from build123d import *

# Parameters (mm, degrees)
SKETCH003_R   = 2
PAD002_DEPTH  = 10
SKETCH_R      = 7
PAD_DEPTH     = 45
SKETCH001_W   = 100
SKETCH001_H   = 10
PAD001_DEPTH  = 5
FILLET_R      = 4.99
SKETCH002_W   = 3
SKETCH002_H   = 13.521623
SKETCH002_H_2 = 14.821778
SKETCH002_H_3 = 14.691763
POCKET_DEPTH  = 4


with BuildPart() as pad002:
    # Sketch003 → Pad002 (new body, symmetric)
    with BuildSketch(Plane(origin=(0, 0, -4), x_dir=(0, 0, -1), z_dir=(1, 0, 0))):
        Circle(SKETCH003_R)
    extrude(amount=PAD002_DEPTH, both=True)


with BuildPart() as cut:
    # Sketch → Pad (new body)
    with BuildSketch(Plane.XY):
        Circle(SKETCH_R)
    extrude(amount=-PAD_DEPTH)

    # Cut: cut Pad002
    add(pad002.part, mode=Mode.SUBTRACT)


with BuildPart() as obj1:
    # Sketch001 → Pad001 (new body, symmetric)
    with BuildSketch(Plane.XY.offset(-45)):
        Rectangle(SKETCH001_W, SKETCH001_H)
    extrude(amount=PAD001_DEPTH, both=True)

    # Fillet
    fillet_edges = [obj1.edges().sort_by_distance(p)[0] for p in [
        (-50, 5, -45),
        (-50, -5, -45),
        (50, 5, -45),
        (50, -5, -45),
    ]]
    fillet(fillet_edges, radius=FILLET_R)

    # Sketch002 → Pocket (cut)
    with BuildSketch(Plane.XY.offset(-40)):
        with Locations((-34.600117, -0.008592)):
            Rectangle(SKETCH002_W, SKETCH002_H)
        with Locations((-14.823811, -0.528653)):
            Rectangle(SKETCH002_W, SKETCH002_H_2)
        with Locations((14.868009, -0.33363)):
            Rectangle(SKETCH002_W, SKETCH002_H_3)
        with Locations((34.916373, -0.463645)):
            Rectangle(SKETCH002_W, SKETCH002_H_3)
    extrude(amount=-POCKET_DEPTH, mode=Mode.SUBTRACT)

    # Fusion: union Cut
    add(cut.part)


solid = obj1.part
Work out the finished part from the listing and answer in its coordinate system (mm). A direction names the side the tool comes from. Coordinates: 2 decimals unless noted, no trailing zeros. Write each loop counter-clockwise with the first axis right and the second up, starting at its lowest first coordinate (ties: lowest second). Pieces come first, ordered by that corner, then holes. Notation, with made-up numbers: M 76,15.25 L 132,15.25 A30 cw 132,45.25 Z; hole C -6,67.5 d5. An arc over 180 degrees is marked long. Answer as CSV lines item,"result". Start each with the question number.
Item 1: Flat-ended cylindrical pins translate along their axes: P1, Ø3, axis at y = 2, z = -42, coming from the -X side; P2, Ø2.5, axis at x = 34.5, y = 1.5, coming from the +Z side; P3, Ø5, axis at y = 0, z = -4, coming from the +X side. Find the tip coordinate at first contact, or state that the pin passes through.
Item 2: Section A-A on x = 0 is taken. Write down the section's boundary in (y, z), and give its area (3 significant figures).
Item 3: Section D-D on z = -4 is taken. Write down the section's boundary in (x, y).
Item 4: Determine the mould class of faces 5 (the face through (48.577, 3.499, -45.07)), 6 (the face through (-15, 0, -44)), 7 (the face through (0, 6, -45)) for opening direction X: released by +X, released by -X, zero draft, split by the parting line, or undercut.
Item 5: Section C-C on z = -18 is taken. Write down the section's boundary in (x, y).
Item 6: Consider L1, parallel to Z at x = -31, y = -0.25; L2, parallel to X at y = -4, z = -41; L3, parallel to Z at x = 6, y = 0. Determine where each line is inside the solid, lowest interval first.
Item 7: Section B-B on y = 1 is taken. Write down the section's boundary in (x, z), and give its area (3 significant figures).
Item 8: A tool of negligible diameter and unlimited length cuts with its end or side. For faces 1 (the face through (-43, 0, -40)), 2 (the face through (0, -6, -45)), 3 (the face through (16.368, 0, -42)), 4 (the face through (43, 0, -40)), from which of +Z, -Z, +X, -X, +Y, -Y can it reach the whole face along a straight path? Write none if from no direction.
Checks:
1,P1,"stops at x = -49.98"
1,P2,"stops at z = -40"
1,P3,"stops at x = 7"
2,outline,"M -7,-45 L -5,-45 L -5,-50 L 5,-50 L 5,-45 L 7,-45 L 7,0 L -7,0 Z; hole C 0,-4 d4"
2,area,"667 mm²"
3,outline,"M -6.71,-2 A7 ccw 6.71,-2 Z; M -6.71,2 L 6.71,2 A7 ccw Z"
4,face 5,"released by +X"
4,face 6,"undercut"
4,face 7,"zero draft"
5,outline,"C 0,0 d14"
6,L1,"z = -50 to -40"
6,L2,"x = -48.01 to -36.1, -33.1 to -16.32, -13.32 to 13.37, 16.37 to 33.42, 36.42 to 48.01"
6,L3,"z = -50 to -6, -2 to 0"
7,outline,"M -49.9,-50 L 49.9,-50 L 49.9,-40 L 36.42,-40 L 36.42,-44 L 33.42,-44 L 33.42,-40 L 16.37,-40 L 16.37,-44 L 13.37,-44 L 13.37,-40 L 6.93,-40 L 6.93,-5.73 L -6.93,-5.73 L -6.93,-40 L -13.32,-40 L -13.32,-44 L -16.32,-44 L -16.32,-40 L -33.1,-40 L -33.1,-44 L -36.1,-44 L -36.1,-40 L -49.9,-40 Z; M -6.93,-2.27 L 6.93,-2.27 L 6.93,0 L -6.93,0 Z"
7,area,"1,460 mm²"
8,face 1,"+Z, -X, +Y, -Y"
8,face 2,"-Z, +X, -X, -Y"
8,face 3,"+Z, +Y, -Y"
8,face 4,"+Z, +X, +Y, -Y"
